```python
from build123d import *

# Parameters (mm, degrees)
SKETCH_1_R          = 28.5
EXTRUDE_1_DEPTH     = 11
SKETCH_3_R          = 18.5
CUT_EXTRUDE_1_DEPTH = 9
SKETCH_4_R          = 17
CUT_EXTRUDE_2_DEPTH = 3
SKETCH_5_R          = 3
CUT_EXTRUDE_3_DEPTH = 12


with BuildPart() as part:
    # 草图1 → 凸台-拉伸1 (new body)
    with BuildSketch(Plane.XY):
        Circle(SKETCH_1_R)
    extrude(amount=EXTRUDE_1_DEPTH)

    # 草图3 → 切除-拉伸1 (cut)
    with BuildSketch(Plane.XY.offset(11)):
        Circle(SKETCH_3_R)
    extrude(amount=-CUT_EXTRUDE_1_DEPTH, mode=Mode.SUBTRACT)

    # 草图4 → 切除-拉伸2 (cut, through all)
    with BuildSketch(Plane.XY.offset(2)):
        Circle(SKETCH_4_R)
    extrude(amount=-CUT_EXTRUDE_2_DEPTH, mode=Mode.SUBTRACT)

    # 草图5 → 切除-拉伸3 (cut, through all)
    with BuildSketch(Plane.XY.offset(11)):
        with Locations((0, 23)):
            Circle(SKETCH_5_R)
        with Locations((19.918584287, -11.5)):
            Circle(SKETCH_5_R)
        with Locations((-19.918584287, -11.5)):
            Circle(SKETCH_5_R)
    extrude(amount=-CUT_EXTRUDE_3_DEPTH, mode=Mode.SUBTRACT)


solid = part.part
```
Can you work these out from the model? Positions are in its coordinate system, mm. A direction names the side the tool comes from. Coordinates: 2 decimals unless noted, no trailing zeros. Write each loop counter-clockwise with the first axis right and the second up, starting at its lowest first coordinate (ties: lowest second). Pieces come first, ordered by that corner, then holes. Notation, with made-up numbers: (66, 68) - (109, 68) arc R25 ccw to (109, 80) - close; hole circle Ø8 at (-1.75, 33). An arc over 180 degrees is marked (long way). Return JSON: item names as keys, results as strings.
Q1. Thinking about a two-plate mould opening in X: for faces 1 (the flat face through (12.3, -12.3, 0)), 2 (the cylindrical face through (-0.65, 20.07, 5.58)), 3 (the cylindrical face through (26.327, -10.916, 5.423)), which applies, +X half, -X half, draft (parallel to the pull), parting line (faces both ways), or undercut?
Computed values:
{"face 1": "draft", "face 2": "undercut", "face 3": "parting line"}
Q2. Please list where these lines run through material, in increasing order: L1, parallel to Y at x = 0, z = 1.2; L2, parallel to Y at x = 0, z = 4.25; L3, parallel to Y at x = -20, z = 0.75. Write a range as from..to.
Computed values:
{"L1": "y = -28.5..-17, 17..20, 26..28.5", "L2": "y = -28.5..-18.5, 18.5..20, 26..28.5", "L3": "y = -20.3..-14.5, -8.5..20.3"}
Q3. If we section it at D-D (x = 10): Please give me the cut outline in (y, z), then the cut area to 3 significant figures.
Computed values:
{"outline": "(-26.69, 0) - (-13.75, 0) - (-13.75, 2) - (-15.56, 2) - (-15.56, 11) - (-26.69, 11) - close; (13.75, 0) - (26.69, 0) - (26.69, 11) - (15.56, 11) - (15.56, 2) - (13.75, 2) - close", "area": "252 mm2"}
Q4. If we section it at C-C (z = 4.5): Please give me the cut outline in (x, y).
Computed values:
{"outline": "circle Ø57 at (0, 0); hole circle Ø6 at (-19.92, -11.5); hole circle Ø37 at (0, 0); hole circle Ø6 at (0, 23); hole circle Ø6 at (19.92, -11.5)"}
Q5. If we section it at A-A (x = 0): Please give me the cut outline in (y, z), then the cut area to 3 significant figures.
Computed values:
{"outline": "(-28.5, 0) - (-17, 0) - (-17, 2) - (-18.5, 2) - (-18.5, 11) - (-28.5, 11) - close; (17, 0) - (20, 0) - (20, 11) - (18.5, 11) - (18.5, 2) - (17, 2) - close; (26, 0) - (28.5, 0) - (28.5, 11) - (26, 11) - close", "area": "160 mm2"}
Q6. On a 3-axis mill with a long thin cutter (end or side, diameter ignored), from which of +Z, -Z, +X, -X, +Y, -Y can I reach the whole of each face in a straight line? I mean faces 4 (the flat face through (5.4, -16.4, 2)), 5 (the cylindrical face through (-17.147, -12.649, 5.577)). Say none if no direction works.
Computed values:
{"face 4": "+Z", "face 5": "+Z, -Z"}
Q7. If we section it at B-B (y = 6.5): Please give me the cut outline in (x, z).
Computed values:
{"outline": "(-27.75, 0) - (-15.71, 0) - (-15.71, 2) - (-17.32, 2) - (-17.32, 11) - (-27.75, 11) - close; (15.71, 0) - (27.75, 0) - (27.75, 11) - (17.32, 11) - (17.32, 2) - (15.71, 2) - close"}
Q8. I'm going to push flat-ended pins straight in: pin 1 Ø1.5 at (x, z) = (-2, 9) entering from +Y; pin 2 Ø8 at (x, y) = (-19, -1) entering from -Z; pin 3 Ø2 at (y, z) = (20, 9.5) entering from +X; pin 4 Ø4 at (x, z) = (-16.5, 2) entering from +Y. Where does each tip first touch, or does it pass through?
Computed values:
{"pin 1": "stops at y = 28.47", "pin 2": "stops at z = 0", "pin 3": "stops at x = 21.24", "pin 4": "stops at y = 24.54"}
